```python
from build123d import *

# Parameters (mm, degrees)
SKETCH_W  = 58
SKETCH_H  = 9.52
SKETCH_R  = 2
PAD_DEPTH = 40
FILLET_R  = 1


with BuildPart() as part:
    # Sketch → Pad (new body)
    with BuildSketch(Plane.XZ):
        Rectangle(SKETCH_W, SKETCH_H)
        with Locations((-23.57, 0)):
            Circle(SKETCH_R, mode=Mode.SUBTRACT)
        with Locations((23.57, 0)):
            Circle(SKETCH_R, mode=Mode.SUBTRACT)
    extrude(amount=PAD_DEPTH)

    # Fillet
    fillet_edges = [part.edges().sort_by_distance(p)[0] for p in [
        (-29, -20, 4.76),
        (29, -20, 4.76),
    ]]
    fillet(fillet_edges, radius=FILLET_R)


solid = part.part
```
Geometry: final body of the model. Coordinates: model frame, mm. Round coordinates to 2 decimals unless told otherwise and drop trailing zeros. Write each loop counter-clockwise with the first axis right and the second up, starting at its lowest first coordinate (ties: lowest second). Pieces come first, ordered by that corner, then holes.
Item 1: Section query B-B (z = 0). Return loops of the section in (x, y), plus the area to 3 significant figures.
Item 2: Material intervals for L1, parallel to Z at x = 23.57, y = -18.5; L2, parallel to X at y = -19, z = -1; L3, parallel to Z at x = 23, y = -20, sorted ascending.
Item 3: Mould query, pull axis Z, two halves, no side actions, for faces 1 (the face through (21.572, -19.72, 0.088)), 2 (the face through (29, -20, -1)), 3 (the face through (0, -20, -4.76)). Classes: +Z half, -Z half, draft (parallel to the pull), parting line (faces both ways), or undercut.
Item 4: Section query A-A (x = -23.57). Return loops of the section in (y, z).
Item 5: Section query C-C (y = -26.5). Return loops of the section in (x, z).
Completed:
1. outline: (-29, -40) - (-25.57, -40) - (-25.57, 0) - (-29, 0) - close; (-21.57, -40) - (21.57, -40) - (21.57, 0) - (-21.57, 0) - close; (25.57, -40) - (29, -40) - (29, 0) - (25.57, 0) - close
1. area: 2,000 mm2
2. L1: z = -4.76 to -2, 2 to 4.76
2. L2: x = -29 to -25.3, -21.84 to 21.84, 25.3 to 29
2. L3: z = -4.76 to -1.92, 1.92 to 4.76
3. face 1: undercut
3. face 2: draft
3. face 3: -Z half
4. outline: (-40, -4.76) - (0, -4.76) - (0, -2) - (-40, -2) - close; (-40, 2) - (0, 2) - (0, 4.76) - (-40, 4.76) - close
5. outline: (-29, -4.76) - (29, -4.76) - (29, 3.76) arc R1 ccw to (28, 4.76) - (-28, 4.76) arc R1 ccw to (-29, 3.76) - close; hole circle Ø4 at (-23.57, 0); hole circle Ø4 at (23.57, 0)
